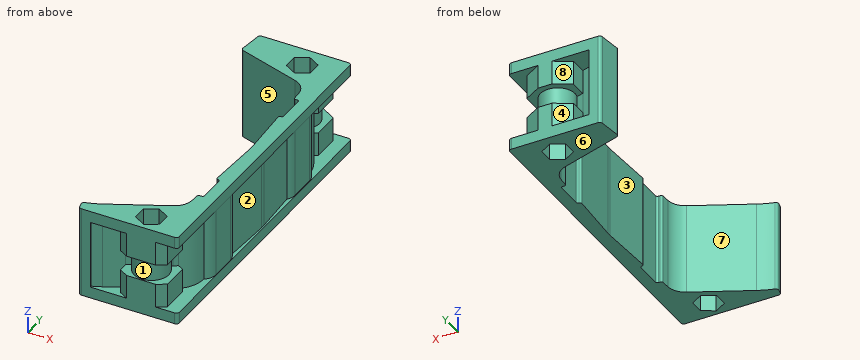
```python
from build123d import *

# Parameters (mm, degrees)
BOSS_EXTRUDE1_DEPTH     = 24.13
CUT_EXTRUDE1_DEPTH      = 138.766550514
CUT_EXTRUDE1_DEPTH_BACK = 138.766550514
FILLET1_R               = 1.5875
CUT_EXTRUDE2_DEPTH      = 12.7
CUT_EXTRUDE3_DEPTH      = 138.766550514
CUT_EXTRUDE3_DEPTH_BACK = 138.766550514
SKETCH4_R               = 3.175
SHELL1_START            = -18.073116
SHELL1_DEPTH            = 36.146232
SHELL1_START_2          = -5.373116
SHELL1_2_DEPTH          = 10.746232


# Read off the part's stored shape, not the designer's step: Shell1
with BuildPart() as part:
    # Sketch1 → Boss-Extrude1 (new, symmetric)
    with BuildSketch(Plane.XY):
        with BuildLine():
            Line((56.161313585, 65.087564001), (56.15, 65.087371974))
            ThreePointArc((56.15, 65.087371974), (55.438759683, 64.766920639), (55.174115771, 64.033084522))
            Line((55.174115771, 64.033084522), (56.680450554, 36.457041128))
            ThreePointArc((56.680450554, 36.457041128), (56.705496383, 35.550244887), (56.681639728, 34.643416582))
            Line((56.681639728, 34.643416582), (55.144848554, 5.815734008))
            ThreePointArc((55.144848554, 5.815734008), (55.417746823, 5.074471658), (56.143430652, 4.7625))
            Line((56.143430652, 4.7625), (56.149999968, 4.762499984))
            ThreePointArc((56.149999968, 4.762499984), (56.857106771, 4.469606766), (57.15, 3.762499968))
            Line((57.15, 3.762499968), (57.15, -10.112499968))
            ThreePointArc((57.15, -10.112499968), (56.857106771, -10.819606766), (56.149999968, -11.112499984))
            Line((56.149999968, -11.112499984), (55.190522202, -11.1125))
            ThreePointArc((55.190522202, -11.1125), (54.502493828, -11.386816202), (54.191940103, -12.059266056))
            Line((54.191940103, -12.059266056), (53.961494186, -16.382053603))
            ThreePointArc((53.961494186, -16.382053603), (52.407837698, -21.109352316), (48.682296217, -24.408070592))
            Line((48.682296217, -24.408070592), (19.327486058, -38.967689038))
            ThreePointArc((19.327486058, -38.967689038), (0, -43.4975), (-19.327486058, -38.967689038))
            Line((-19.327486058, -38.967689038), (-19.327486058, -47.388950103))
            Line((-19.327486058, -47.388950103), (63.5, -47.388950103))
            Line((63.5, -47.388950103), (63.5, 119.854559949))
            Line((63.5, 119.854559949), (-4.702524006, 119.854559949))
            Line((-4.702524006, 119.854559949), (-4.702524006, 108.02491605))
            ThreePointArc((-4.702524006, 108.02491605), (0, 108.7374), (4.702524006, 108.02491605))
            Line((4.702524006, 108.02491605), (47.271514403, 94.82250963))
            ThreePointArc((47.271514403, 94.82250963), (51.961130003, 91.582350175), (53.960821068, 86.244526329))
            Line((53.960821068, 86.244526329), (54.197705155, 81.907956584))
            ThreePointArc((54.197705155, 81.907956584), (54.508664182, 81.236365226), (55.196216585, 80.9625))
            Line((55.196216585, 80.9625), (56.149999984, 80.962499984))
            ThreePointArc((56.149999984, 80.962499984), (56.857106777, 80.669606761), (57.15, 79.962499968))
            Line((57.15, 79.962499968), (57.15, 66.087500032))
            ThreePointArc((57.15, 66.087500032), (56.8610955, 65.384404568), (56.161313585, 65.087564001))
        make_face()
    extrude(amount=BOSS_EXTRUDE1_DEPTH, both=True)

    # Sketch2 → Cut-Extrude1 (cut, two sides: drawn at the far end of the back side and taken through both)
    with BuildSketch(Plane.XY.offset(-CUT_EXTRUDE1_DEPTH_BACK)):
        Polygon((0, 0), (16.649604997, 137.747881839), (-33.336773011, 132.313158031), (-32.126746787, -67.704176811), (15.765326083, -67.704176811), align=None)
    extrude(amount=CUT_EXTRUDE1_DEPTH + CUT_EXTRUDE1_DEPTH_BACK, mode=Mode.SUBTRACT)

    # Fillet1
    fillet1_edges = [part.edges().sort_by_distance(p)[0] for p in [
        (63.5, 119.854559949, 0),
        (63.5, -47.388950103, 0),
        (11.034802966, -47.388950103, 0),
        (9.864742858, -42.364128158, 0),
        (12.755119811, 105.527472687, 0),
        (14.486836775, 119.854559949, 0),
    ]]
    fillet(fillet1_edges, radius=FILLET1_R)

    # Sketch3 → Cut-Extrude2 (cut)
    with BuildSketch(Plane(origin=(0, 0, -24.13), x_dir=(-1, 0, 0), z_dir=(0, 0, -1))):
        Polygon((-44.059380862, -30.050777043), (-50.460180862, -33.746280646), (-50.460180862, -41.137287852), (-44.059380862, -44.832791455), (-37.658580862, -41.137287852), (-37.658580862, -33.746280646), align=None)
        Polygon((-37.658580862, 111.2671939), (-44.059380862, 114.962697503), (-50.460180862, 111.2671939), (-50.460180862, 103.876186694), (-44.059380862, 100.180683091), (-37.658580862, 103.876186694), align=None)
    cut_extrude2 = extrude(amount=-CUT_EXTRUDE2_DEPTH, mode=Mode.SUBTRACT)

    # Mirror1: Cut-Extrude2 across plane
    add(cut_extrude2.mirror(Plane.XY), mode=Mode.SUBTRACT)

    # Sketch4 → Cut-Extrude3 (cut, two sides: drawn at the far end of the back side and taken through both)
    with BuildSketch(Plane.XY.offset(-CUT_EXTRUDE3_DEPTH_BACK)):
        with Locations((44.059380862, 107.571690297)):
            Circle(SKETCH4_R)
        with Locations((44.059380862, -37.441784249)):
            Circle(SKETCH4_R)
    extrude(amount=CUT_EXTRUDE3_DEPTH + CUT_EXTRUDE3_DEPTH_BACK, mode=Mode.SUBTRACT)

    # Shell1 outline → Shell1 (cut)
    with BuildSketch(Plane.XY.offset(SHELL1_START)):
        with BuildLine():
            ThreePointArc((60.031332227, -16.006129752), (58.284234513, -23.045011467), (53.540141007, -28.530609249))
            Line((53.540141007, -28.530609249), (56.517064862, -30.249337038))
            Line((56.517064862, -30.249337038), (56.517064862, -44.63423146))
            Line((56.517064862, -44.63423146), (51.745752212, -47.388950103))
            Line((51.745752212, -47.388950103), (61.9125, -47.388950103))
            ThreePointArc((61.9125, -47.388950103), (63.035032015, -46.923982118), (63.5, -45.801450103))
            Line((63.5, -45.801450103), (63.5, 118.267059949))
            ThreePointArc((63.5, 118.267059949), (63.035032015, 119.389591964), (61.9125, 119.854559949))
            Line((61.9125, 119.854559949), (47.700194563, 119.854559949))
            Line((47.700194563, 119.854559949), (56.517064862, 114.764137508))
            Line((56.517064862, 114.764137508), (56.517064862, 100.379243086))
            Line((56.517064862, 100.379243086), (53.321926303, 98.534528979))
            ThreePointArc((53.321926303, 98.534528979), (58.222287934, 93.013291574), (60.031332227, 85.856129752))
            ThreePointArc((60.031332227, 85.856129752), (62.362476281, 83.309849707), (63.206884, 79.962499968))
            Line((63.206884, 79.962499968), (63.206884008, 66.087500032))
            ThreePointArc((63.206884008, 66.087500032), (62.736011515, 63.552926254), (61.386232226, 61.356592716))
            Line((61.386232226, 61.356592716), (62.728318266, 36.787404457))
            ThreePointArc((62.728318266, 36.787404457), (62.762379081, 35.55421632), (62.729935471, 34.320984576))
            Line((62.729935471, 34.320984576), (61.354914269, 8.527841436))
            ThreePointArc((61.354914269, 8.527841436), (62.727616894, 6.318780038), (63.206884, 3.762499968))
            Line((63.206884, 3.762499968), (63.206884, -10.112499968))
            ThreePointArc((63.206884, -10.112499968), (62.362476281, -13.459849707), (60.031332227, -16.006129752))
        make_face()
        with BuildLine():
            Line((31.601696862, -44.63423146), (31.601696862, -39.640802436))
            Line((31.601696862, -39.640802436), (22.018775007, -44.39381174))
            ThreePointArc((22.018775007, -44.39381174), (19.565089882, -45.528499114), (17.053178169, -46.527691625))
            Line((17.053178169, -46.527691625), (17.253727402, -47.388950103))
            Line((17.253727402, -47.388950103), (36.373009512, -47.388950103))
            Line((36.373009512, -47.388950103), (31.601696862, -44.63423146))
        make_face()
        Polygon((31.601696862, 114.764137508), (40.418567161, 119.854559949), (20.587804641, 119.854559949), (19.374447508, 109.816041015), (31.601696862, 106.023864741), align=None)
    extrude(amount=SHELL1_DEPTH, mode=Mode.SUBTRACT)

    # Shell1 2 outline → Shell1 2 (cut)
    with BuildSketch(Plane.XY.offset(SHELL1_START_2)):
        with BuildLine():
            ThreePointArc((53.540141007, -28.530609249), (52.483348575, -29.226420137), (51.373585166, -29.834193295))
            Line((51.373585166, -29.834193295), (50.103961944, -30.463910523))
            ThreePointArc((50.103961944, -30.463910523), (48.161435217, -45.712263816), (34.846350755, -38.031494714))
            Line((34.846350755, -38.031494714), (31.601696862, -39.640802436))
            Line((31.601696862, -39.640802436), (31.601696862, -44.63423146))
            Line((31.601696862, -44.63423146), (36.373009512, -47.388950103))
            Line((36.373009512, -47.388950103), (51.745752212, -47.388950103))
            Line((51.745752212, -47.388950103), (56.517064862, -44.63423146))
            Line((56.517064862, -44.63423146), (56.517064862, -30.249337038))
            Line((56.517064862, -30.249337038), (53.540141007, -28.530609249))
        make_face()
        with BuildLine():
            Line((56.517064862, 114.764137508), (47.700194563, 119.854559949))
            Line((47.700194563, 119.854559949), (40.418567161, 119.854559949))
            Line((40.418567161, 119.854559949), (31.601696862, 114.764137508))
            Line((31.601696862, 114.764137508), (31.601696862, 106.023864741))
            Line((31.601696862, 106.023864741), (35.222242894, 104.900983514))
            ThreePointArc((35.222242894, 104.900983514), (46.805661297, 116.385635269), (49.81545048, 100.353979805))
            ThreePointArc((49.81545048, 100.353979805), (51.626581689, 99.555827316), (53.321926303, 98.534528979))
            Line((53.321926303, 98.534528979), (56.517064862, 100.379243086))
            Line((56.517064862, 100.379243086), (56.517064862, 114.764137508))
        make_face()
    extrude(amount=SHELL1_2_DEPTH, mode=Mode.SUBTRACT)


solid = part.part
```
Input: part model. Units: mm. Frame: model coordinates. Face numbers are marked on the shaded views. A direction names the side the tool comes from. Round coordinates to 2 decimals unless told otherwise and drop trailing zeros. Order: outer loops, then holes, each group sorted by start corner. A loop starts at its lowest first (then second) coordinate and runs counter-clockwise, first axis right, second up. Notation, with made-up numbers: (68.25, -11) - (94.25, -11) arc R20 cw to (94.25, 3) - close; hole circle Ø5 at (-13, -12). An arc over 180 degrees is marked (long way). One line per question, with ' | ' between items. Start each with the question number.
1) Contact query for flat-ended pins moving along their axis: P1, Ø1, axis at x = 56, z = 0.5, coming from the -Y side; P2, Ø6, axis at x = 57, z = 2, coming from the +Y side; P3, Ø2, axis at x = 27, z = -12, coming from the +Y side; P4, Ø1.5, axis at y = 30.5, z = 17.5, coming from the +X side. Output: stop coordinate, or through.
2) Pull-direction query (Y, two-part tool) for the marked faces 5, 6, 7 and 8; classes: +Y half, -Y half, draft (parallel to the pull), parting line (faces both ways), or undercut.
3) Set-up query: the marked faces 1, 2, 3 and 4. Return all of +Z, -Z, +X, -X, +Y, -Y with unobstructed straight access to the full face (end or side cutting, diameter ignored); none if empty.
4) Cut plane B-B, the plane z = -20. Give the number of separate pieces and of enclosed holes in the cut face, then the cut area to 3 significant figures.
5) Cut plane C-C, the plane y = 54. Return the cut outline in (x, z), then the cut area to 3 significant figures.
6) Ray query, probe 1 along Z at (x, y) = (39, 111.5); probe 2 along Y at (x, z) = (43, 17); probe 3 along Y at (x, z) = (27.5, -17). Return the intervals inside material, ascending.
7) Cut plane A-A, the plane y = 77. Return the cut outline in (x, z).
Worked out:
1) P1: stops at y = -26.86 | P2: stops at y = 98.04 | P3: stops at y = 107.76 | P4: stops at x = 63.5
2) face 5: undercut | face 6: draft | face 7: undercut | face 8: +Y half
3) face 1: none | face 2: +X | face 3: +Z, -Z, -X | face 4: +Y
4) separate pieces: 1 | enclosed holes: 2 | area: 2,590 mm^2
5) outline: (55.72, -24.13) - (63.5, -24.13) - (63.5, -18.07) - (61.79, -18.07) - (61.79, 18.07) - (63.5, 18.07) - (63.5, 24.13) - (55.72, 24.13) - close | area: 313 mm^2
6) probe 1: z = -11.43 to 11.43 | probe 2: y = -47.39 to -44.22, -30.66 to -27.23, 96.15 to 100.79, 114.35 to 119.85 | probe 3: y = -41.68 to -34.91, 100.95 to 107.3
7) outline: (57.15, -24.13) - (63.5, -24.13) - (63.5, -18.07) - (63.21, -18.07) - (63.21, 18.07) - (63.5, 18.07) - (63.5, 24.13) - (57.15, 24.13) - close
